Source: CAD feature listing. Evaluate the final solid. Frame: model axes, mm. A direction names the side the tool comes from. Give positions to 0.01 mm unless a question says otherwise; leave off trailing zeros. Order: outer loops, then holes, each group sorted by start corner. A loop starts at its lowest first (then second) coordinate and runs counter-clockwise, first axis right, second up. Notation, with made-up numbers: M 35.5,-25.5 L 90.5,-25.5 A16 ccw 90.5,-16.5 Z; hole C -35,64 d6. An arc over 180 degrees is marked long. Answer as a JSON object with one key per item and string values. Group by question number.
1. Section query D-D (z = -102). Output: boundary loops of the cut face in (x, y), plus the area to 3 significant figures.
2. Section query C-C (z = -78). Output: boundary loops of the cut face in (x, y).
3. Material intervals for L1, parallel to Z at x = -76, y = 26; L2, parallel to Y at x = 32, z = -89; L3, parallel to Z at x = 44.5, y = 94.5, sorted ascending. Write a range as [from, to].
4. Set-up query: faces 5 (the flat face through (-2, 30, 0)), 6 (the flat face through (9.5, 77, -26)), 7 (the flat face through (-10.5, 78, -27)), 8 (the flat face through (-0.13, 85.37, -32.54)), 9 (the flat face through (-2, 30, -1)). Return all of +Z, -Z, +X, -X, +Y, -Y with unobstructed straight access to the full face (end or side cutting, diameter ignored); none if empty.
5. Section query B-B (x = -24.5). Output: boundary loops of the cut face in (y, z).
6. Pull-direction query (Z, two-part tool) for faces 1 (the flat face through (0.15, 85.81, -33.78)), 2 (the flat face through (-0.133, 72.775, -35.088)), 3 (the flat face through (2, 98.302, -62)), 4 (the flat face through (2.1, 70.37, -8.7)); classes: +Z half, -Z half, draft (parallel to the pull), parting line (faces both ways), or undercut.
7. Section query A-A (y = 55.5). Output: boundary loops of the cut face in (x, z).
8. Pin query (flat end, axial travel): P1, Ø12.5, axis at y = 76.5, z = -30.5, coming from the +X side; P2, Ø21.5, axis at y = 73.5, z = -22.5, coming from the -X side; P3, Ø6, axis at x = -65.5, z = -22, coming from the -Y side; P4, Ø7.5, axis at y = 71.5, z = -32.5, coming from the -X side. Return the tip coordinate at first contact, or that it passes through.
from build123d import *

# Parameters (mm, degrees)
SKETCH_1_W          = 300
SKETCH_1_H          = 60
EXTRUDE_1_DEPTH     = 1
SKETCH_4_W          = 300
SKETCH_4_H          = 1.002930946
EXTRUDE_2_DEPTH     = 50
SKETCH_5_W          = 300
SKETCH_5_H          = 1.001378412
EXTRUDE_3_DEPTH     = 60
SKETCH_11_W         = 21
SKETCH_11_H         = 21
EXTRUDE_5_DEPTH     = 25
SHELL_START         = -9.5
SHELL_1_DEPTH       = 19
SHELL_START_2       = -10.5
SHELL_1_2_DEPTH     = 21
SKETCH_12_R         = 8.5
CUT_EXTRUDE_4_DEPTH = 1


# Read off the part's stored shape, not the designer's step: 抽壳1
with BuildPart() as part:
    # 草图1 → 凸台-拉伸1 (new body)
    with BuildSketch(Plane.XY):
        with Locations((0, 30)):
            Rectangle(SKETCH_1_W, SKETCH_1_H)
    extrude_1 = extrude(amount=-EXTRUDE_1_DEPTH)

    # 草图4 → 凸台-拉伸2 (add)
    with BuildSketch(Plane(origin=(0, 35.20944533, -29.54423259), x_dir=(-1, 0, 0), z_dir=(0, 0.7660444431189771, -0.6427876096865406))):
        with Locations((0, 38.065791108)):
            Rectangle(SKETCH_4_W, SKETCH_4_H)
    extrude_2 = extrude(amount=EXTRUDE_2_DEPTH)

    # 草图5 → 凸台-拉伸3 (add)
    with BuildSketch(Plane(origin=(0, 0, -32.139380484), x_dir=(-1, 0, 0), z_dir=(0, 0, -1))):
        with Locations((0, 97.80153295)):
            Rectangle(SKETCH_5_W, SKETCH_5_H)
    extrude(amount=EXTRUDE_3_DEPTH)

    # 镜向1: 凸台-拉伸2 across plane
    add(extrude_2.mirror(Plane.XY.offset(-62.139380484)))

    # 镜向2: 凸台-拉伸1 across plane
    add(extrude_1.mirror(Plane.XY.offset(-62.139380484)))

    # 草图11 → 凸台-拉伸5 (add)
    with BuildSketch(Plane(origin=(0, 15, 25.980762114), x_dir=(-1, 0, 0), z_dir=(0, 0.500000000000001, 0.8660254037844382))):
        with Locations((0, -80.701911878)):
            Rectangle(SKETCH_11_W, SKETCH_11_H)
    extrude(amount=-EXTRUDE_5_DEPTH)

    # 抽壳1 outline → 抽壳1 (cut)
    with BuildSketch(Plane.YZ.offset(SHELL_START)):
        Polygon((89.744253028, -24.962217823), (90.522114942, -25.614921468), (90.523603022, -25.612344038), (93.98317256, -19.620193825), (75.79663908, -9.120193825), (74.18850284, -11.9055675), (74.187014759, -11.90814493), (74.964876673, -12.560848575), (64.662664484, -30.404803516), (81.117147156, -39.904803516), align=None)
    extrude(amount=SHELL_1_DEPTH, mode=Mode.SUBTRACT)

    # Shell 1 2 outline → Shell 1 2 (cut)
    with BuildSketch(Plane.YZ.offset(SHELL_START_2)):
        Polygon((74.187014759, -11.90814493), (90.522114942, -25.614921468), (90.523603022, -25.612344038), (93.98317256, -19.620193825), (75.79663908, -9.120193825), (74.18850284, -11.9055675), align=None)
    extrude(amount=SHELL_1_2_DEPTH, mode=Mode.SUBTRACT)

    # 草图12 → 切除-拉伸4 (cut)
    with BuildSketch(Plane(origin=(0, 60.79663908, -35.100955939), x_dir=(1, 0, 0), z_dir=(0, -0.8660254037844382, 0.5000000000000011))):
        with Locations(Location((0, 14, 0), (0, 0, 270))):
            Circle(SKETCH_12_R)
    extrude(amount=-CUT_EXTRUDE_4_DEPTH, mode=Mode.SUBTRACT)


solid = part.part
Answer sheet:
{
 "1": {"outline": "M -150,84.99 L 150,84.99 L 150,86.55 L -150,86.55 Z", "area": "468 mm^2"},
 "2": {"outline": "M -150,97.3 L 150,97.3 L 150,98.3 L -150,98.3 Z"},
 "3": {"L1": "[-124.28, -123.28], [-1, 0]", "L2": "[97.3, 98.3]", "L3": "[-95.33, -94.02], [-30.26, -28.95]"},
 "4": {"face 5": "+Z, +X, -X, +Y, -Y", "face 6": "none", "face 7": "-X, -Y", "face 8": "+Z", "face 9": "+X, -X, -Y"},
 "5": {"outline": "M 0,-124.28 L 60,-124.28 L 98.3,-92.14 L 98.3,-32.14 L 60,0 L 0,0 L 0,-1 L 59.63,-1 L 97.3,-32.61 L 97.3,-91.67 L 59.63,-123.28 L 0,-123.28 Z"},
 "6": {"face 1": "undercut", "face 2": "undercut", "face 3": "draft", "face 4": "+Z half"},
 "7": {"outline": "M -150,-124.28 L 150,-124.28 L 150,-123.28 L -150,-123.28 Z; M -150,-1 L 150,-1 L 150,0 L -150,0 Z"},
 "8": {"P1": "x = 10.5", "P2": "x = -150", "P3": "y = 81.08", "P4": "x = -10.5"}
}
